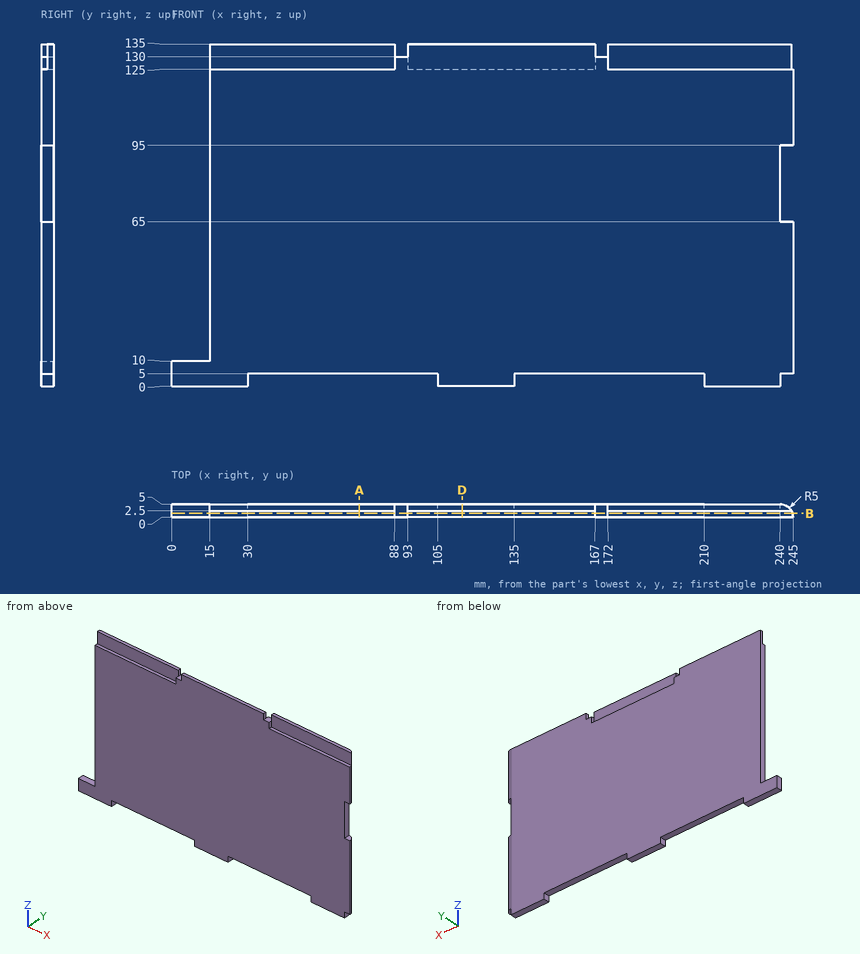
Verification items for this drawing (mm, ordinates from the low corner). Round coordinates to 2 decimals unless told otherwise and drop trailing zeros. Loops run counter-clockwise (first coordinate to the right, second up) from the corner with the lowest first, then second, coordinate; pieces in that order, holes last. Notation, with made-up numbers: (53.25, 2.25) -> (81.25, 2.25) arc R23 ccw to (81.25, 17.25) -> close; hole circle Ø1 at (-15.5, 19.5). An arc over 180 degrees is marked (long way). Answer in a Markdown table with one row per item.
Q1. Thickness scan on L1, parallel to Y at x = 129, z = 127.5; L2, parallel to Z at x = 32.5, y = 2.45; L3, parallel to Z at x = 169, y = 0.7. Record the ranges inside material, lowest first.
Data:
| item | result |
|---|---|
| L1 | y = 0 to 2.5 |
| L2 | z = 5 to 125 |
| L3 | z = 5 to 130 |
Q2. Sectioned sample at B-B on y = 1.4. Enter the section's corners in (x, z), then the cut area to 3 significant figures.
Data:
| item | result |
|---|---|
| outline | (0, 0) -> (30, 0) -> (30, 5) -> (105, 5) -> (105, 0) -> (135, 0) -> (135, 5) -> (210, 5) -> (210, 0) -> (240, 0) -> (240, 5) -> (244.8, 5) -> (244.8, 65) -> (240, 65) -> (240, 95) -> (244.8, 95) -> (244.8, 125) -> (172, 125) -> (172, 130) -> (167, 130) -> (167, 135) -> (93, 135) -> (93, 130) -> (88, 130) -> (88, 125) -> (15, 125) -> (15, 10) -> (0, 10) -> close |
| area | 28,700 mm^2 |
Q3. Sectioned sample at D-D on x = 114.5. Enter the section's corners in (y, z), then the cut area to 3 significant figures.
Data:
| item | result |
|---|---|
| outline | (0, 0) -> (5, 0) -> (5, 125) -> (2.5, 125) -> (2.5, 135) -> (0, 135) -> close |
| area | 650 mm^2 |
Q4. Go/stop test with flat-tipped pins: P1, Ø11, axis at x = 127, z = 127.5, coming from the +Y side; P2, Ø1.2, axis at y = 1, z = 127.5, coming from the +X side; P3, Ø3, axis at x = 220.5, y = 0.5, coming from the +Z side; P4, Ø0.8, axis at y = 3.5, z = 128.5, coming from the +X side. Record where each tip stops, or that it passes through.
Data:
| item | result |
|---|---|
| P1 | stops at y = 5 |
| P2 | stops at x = 172 |
| P3 | stops at z = 125 |
| P4 | stops at x = 243.92 |
Q5. Sectioned sample at A-A on x = 74. Enter the section's corners in (y, z).
Data:
| item | result |
|---|---|
| outline | (0, 5) -> (5, 5) -> (5, 135) -> (2.5, 135) -> (2.5, 125) -> (0, 125) -> close |
